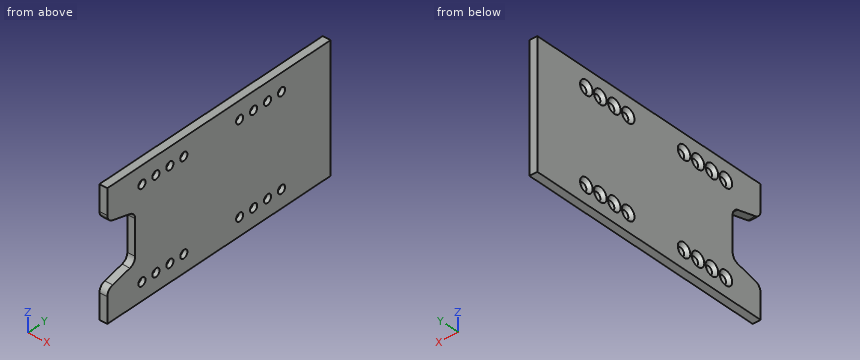
Autodesk Inventor part; units mm, degrees
ref_plane "YZ Plane" through (0, 0, 0) normal (1, 0, 0) x (0, 1, 0)
ref_plane "XZ Plane" through (0, 0, 0) normal (0, 1, 0) x (-1, 0, 0)
ref_plane "XY Plane" through (0, 0, 0) normal (0, 0, 1) x (1, 0, 0)
sketch "Sketch1" plane through (0, 0, 0) normal (1, 0, 0) x (0, 1, 0)
  line L0 (50.8, 25.4) -> (-50.8, 25.4)
  line L1 (-50.8, 25.4) -> (-50.8, -25.4)
  line L2 (-50.8, -25.4) -> (50.8, -25.4)
  line L3 (50.8, -25.4) -> (50.8, 25.4)
  line L4 (50.8, 25.4) -> (-50.8, -25.4) construction
  line L5 (-50.8, 25.4) -> (50.8, -25.4) construction
  line L6 (0, 0) -> (-50.8, 0) construction
  line L7 (-38.1, -9.525) -> (-50.8, -9.525)
  line L8 (-50.8, -9.525) -> (-50.8, 9.525)
  line L9 (-50.8, 9.525) -> (-38.1, 9.525)
  line L10 (-38.1, 9.525) -> (-38.1, -9.525)
  line L11 (-38.1, -9.525) -> (-50.8, 9.525) construction
  line L12 (-50.8, -9.525) -> (-38.1, 9.525) construction
  line L13 (-38.1, -9.525) -> (-50.8, -12.7)
  line L14 (-38.1, 9.525) -> (-50.8, 12.7)
  line L15 (0, -25.4) -> (0, 25.4) construction
  line L16 (38.1, -9.525) -> (50.8, -9.525) construction
  line L17 (50.8, -9.525) -> (50.8, 9.525)
  line L18 (50.8, 9.525) -> (38.1, 9.525) construction
  line L19 (38.1, 9.525) -> (38.1, -9.525)
  line L20 (38.1, -9.525) -> (50.8, 9.525) construction
  line L21 (50.8, -9.525) -> (38.1, 9.525) construction
  line L22 (38.1, -9.525) -> (50.8, -12.7)
  line L23 (38.1, 9.525) -> (50.8, 12.7)
  point P0 (-44.45, 0)
  point P1 (50.8, 0)
  point P2 (44.45, 0)
  point P3 (50.8, -12.7)
  dimension "d0" = 101.6
  dimension "d1" = 50.8
  dimension "d19" = 12.7
  dimension "d20" = 19.05
  dimension "d21" = 12.7
extrude "Extrusion1" add sketch "Sketch1" along normal blind 3.175 contours L3 L23 L19 L22 L2 L1 L13 L10 L14 L0 | L3 L22 L19 L23
fillet "Fillet2" radius 3.175 4 edges at (1.5875, -38.1, 9.525) (1.5875, -50.8, 12.7) (1.5875, -38.1, -9.525) (1.5875, -50.8, -12.7)
sketch "Sketch5" plane through (0, 0, 0) normal (-1, 0, 0) x (0, 0, 1)
  point P0 (18.2563, -35.0209)
  point P1 (18.2563, -28.6709)
  point P2 (18.2563, -22.3209)
  point P3 (18.2563, -15.9709)
  point P4 (18.2563, 9.4291)
  point P5 (18.2563, 15.7791)
  point P6 (18.2563, 22.1291)
  point P7 (18.2563, 28.4791)
  point P8 (-18.2562, 28.4791)
  point P9 (-18.2562, 22.1291)
  point P10 (-18.2562, 15.7791)
  point P11 (-18.2562, 9.4291)
  point P12 (-18.2562, -15.9709)
  point P13 (-18.2562, -22.3209)
  point P14 (-18.2562, -28.6709)
  point P15 (-18.2562, -35.0209)
hole "Hole3" at (0, -35.0209, 18.2563) at (0, -28.6709, 18.2563) at (0, -22.3209, 18.2563) at (0, -15.9709, 18.2563) at (0, 9.4291, 18.2563) at (0, 15.7791, 18.2563) at (0, 22.1291, 18.2563) at (0, 28.4791, 18.2563) at (0, 28.4791, -18.2562) at (0, 22.1291, -18.2562) at (0, 15.7791, -18.2562) at (0, 9.4291, -18.2562) at (0, -15.9709, -18.2562) at (0, -22.3209, -18.2562) at (0, -28.6709, -18.2562) at (0, -35.0209, -18.2562) direction (1, 0, 0) diameter 3.2639 end through all countersink diameter 5.715 countersink angle 82
properties part number "Ramp" material "UHMW, White"
Read the model definition and answer for the solid it produces. Units are mm, in the model's axes. Give positions to 0.01 mm unless a question says otherwise; leave off trailing zeros. Write each loop counter-clockwise with the first axis right and the second up, starting at its lowest first coordinate (ties: lowest second). Pieces come first, ordered by that corner, then holes. Notation, with made-up numbers: (-19.75, -30.5) - (28.25, -30.5) arc R31 ccw to (28.25, -4.5) - close; hole circle Ø11 at (38.25, 63). An arc over 180 degrees is marked (long way). Write item = value, one per line. Start each with the question number.
Item 1: Find the intervals of material crossed by probe 1 along Z at (x, y) = (1.6, -30); probe 2 along Z at (x, y) = (0.7, 29.5); probe 3 along Z at (x, y) = (1.2, -45), in increasing order. Write a range as [from, to].
Item 2: Each of these flat-tipped pins is pushed along its axis until it touches: P1, Ø3, axis at y = 9.43, z = -18.26, coming from the +X side; P2, Ø5, axis at y = -15.97, z = -18.26, coming from the -X side; P3, Ø4, axis at y = 28.48, z = 18.26, coming from the -X side. Where does it stop, or does it pass through?
Item 3: Find section A-A (x = 2.3). State how many separate pieces and enclosed holes the cut face has, then the cut area to 3 significant figures.
Item 4: Find section C-C (z = -8.5). Give the vertices of the cut face in (x, y) (3 decimals).
Item 5: Find section B-B (z = 5.5). Give the vertices of the cut face in (x, y) (3 decimals).
Response:
q1.probe_1 = [-25.4, -19.2], [-17.31, 17.31], [19.2, 25.4]
q1.probe_2 = [-25.4, -20.26], [-16.25, 16.25], [20.26, 25.4]
q1.probe_3 = [-25.4, -11.25], [11.25, 25.4]
q2.P1 = through
q2.P2 = 0.41
q2.P3 = 0.98
q3.separate_pieces = 1
q3.enclosed_holes = 16
q3.area = 4,750 mm²
q4.outline = (0, -38.452) - (3.175, -38.452) - (3.175, 50.8) - (0, 50.8) - close
q5.outline = (0, -38.1) - (3.175, -38.1) - (3.175, 50.8) - (0, 50.8) - close
